Source: CAD feature listing. Evaluate the final solid. Frame: model axes, mm. Face numbers are marked on the shaded views. Round coordinates to 2 decimals unless told otherwise and drop trailing zeros. Loops run counter-clockwise (first coordinate to the right, second up) from the corner with the lowest first, then second, coordinate; pieces in that order, holes last. Notation, with made-up numbers: (-23, 86.25) -> (-13, 86.25) arc R5 ccw to (-13, 94.25) -> close; hole circle Ø11 at (47.5, 33.25). An arc over 180 degrees is marked (long way). Write item = value, one per line.
from build123d import *

# Parameters (mm, degrees)
SKETCH1_W           = 17.018
SKETCH1_H           = 7.62
BOSS_EXTRUDE1_DEPTH = 3.81
FILLET1_R           = 1.27
CUT_EXTRUDE8_REACH  = 37.332
CUT_EXTRUDE9_REACH  = 39.597
SKETCH4_R           = 1.778


with BuildPart() as part:
    # Sketch1 → Boss-Extrude1 (new body)
    with BuildSketch(Plane.XY):
        with Locations((-25.78059107, -11.13155)):
            Rectangle(SKETCH1_W, SKETCH1_H)
    extrude(amount=BOSS_EXTRUDE1_DEPTH)

    # Fillet1
    fillet1_edges = [part.edges().sort_by_distance(p)[0] for p in [
        (-17.27159107, -11.13155, 3.81),
        (-25.78059107, -14.94155, 3.81),
        (-34.28959107, -7.32155, 1.905),
        (-17.27159107, -7.32155, 1.905),
        (-17.27159107, -14.94155, 1.905),
    ]]
    fillet(fillet1_edges, radius=FILLET1_R)

    # Sketch3 → Cut-Extrude8 (cut, up to next)
    with BuildSketch(Plane.XZ.offset(14.94155), mode=Mode.PRIVATE) as cut_extrude8_sk1:
        with BuildLine():
            Line((-23.87560377, 0), (-23.87560377, 1.01854))
            ThreePointArc((-23.87560377, 1.01854), (-24.89159107, 2.0345273), (-25.90757837, 1.01854))
            Line((-25.90757837, 1.01854), (-25.90757837, 0))
            Line((-25.90757837, 0), (-23.87560377, 0))
        make_face()
    cut_extrude8_tool1 = extrude(cut_extrude8_sk1.sketch, amount=-CUT_EXTRUDE8_REACH, mode=Mode.PRIVATE) & part.part
    add(cut_extrude8_tool1.solids().sort_by_distance((-24.891591, -14.94155, 0.922401))[0], mode=Mode.SUBTRACT)

    # Sketch4 → Cut-Extrude9 (cut, up to next)
    with BuildSketch(Plane.XY.offset(3.81), mode=Mode.PRIVATE) as cut_extrude9_sk1:
        with Locations((-20.06559107, -11.13155)):
            Circle(SKETCH4_R)
    cut_extrude9_tool1 = extrude(cut_extrude9_sk1.sketch, amount=-CUT_EXTRUDE9_REACH, mode=Mode.PRIVATE) & part.part
    add(cut_extrude9_tool1.solids().sort_by_distance((-20.065591, -11.13155, 3.81))[0], mode=Mode.SUBTRACT)


solid = part.part
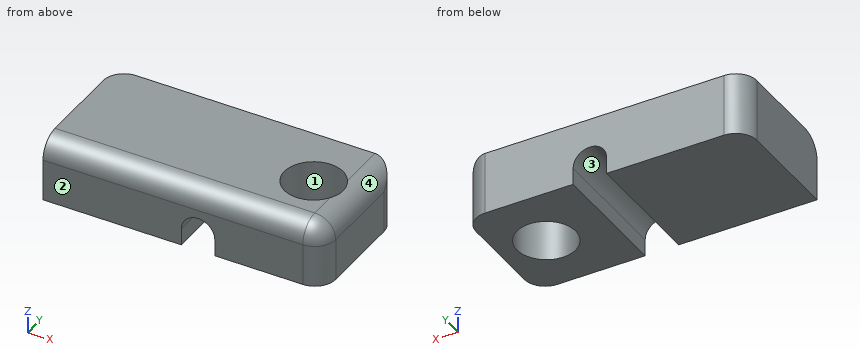
1. Mould query, pull axis X, two halves, no side actions, for the marked faces 1, 2, 3 and 4. Classes: released by +X, released by -X, zero draft, split by the parting line, or undercut.
Evaluation:
face_1 = undercut
face_2 = zero draft
face_3 = undercut
face_4 = released by +X
2. Line query: probe 1 along X at (y, z) = (-11.5, 1.25) (3 decimals); probe 2 along X at (y, z) = (-14.5, 0.4); probe 3 along X at (y, z) = (-14.5, 1.85). Output: solid intervals per line, ascending. Write a range as from..to.
Evaluation:
probe_1 = -34.29..-25.881, -23.902..-21.805, -18.326..-17.272
probe_2 = -34.29..-25.91, -23.88..-17.58
probe_3 = -34.29..-25.48, -24.31..-17.58
3. Section query B-B (y = -10.5). Return the cut outline in (x, z).
Evaluation:
outline = (-34.29, 0) -> (-25.91, 0) -> (-25.91, 1.02) arc R1.02 cw to (-23.88, 1.02) -> (-23.88, 0) -> (-21.73, 0) -> (-21.73, 3.81) -> (-34.29, 3.81) -> close; (-18.4, 0) -> (-17.27, 0) -> (-17.27, 2.54) arc R1.27 ccw to (-18.4, 3.8) -> close
4. Section query D-D (y = -13.25). Return the cut outline in (x, z), then the cut area to 3 significant figures.
Evaluation:
outline = (-34.29, 0) -> (-25.91, 0) -> (-25.91, 1.02) arc R1.02 cw to (-23.88, 1.02) -> (-23.88, 0) -> (-17.27, 0) -> (-17.27, 2.54) arc R1.27 ccw to (-18.54, 3.81) -> (-34.29, 3.81) -> close
area = 60.8 mm²
5. Section query A-A (z = 0.5). Return the cut outline in (x, y).
Evaluation:
outline = (-34.29, -14.94) -> (-25.91, -14.94) -> (-25.91, -7.32) -> (-33.02, -7.32) arc R1.27 ccw to (-34.29, -8.59) -> close; (-23.88, -14.94) -> (-18.54, -14.94) arc R1.27 ccw to (-17.27, -13.67) -> (-17.27, -8.59) arc R1.27 ccw to (-18.54, -7.32) -> (-23.88, -7.32) -> close; hole circle Ø3.56 at (-20.07, -11.13)
6. Section query C-C (x = -21.5). Return the cut outline in (y, z), then the cut area to 3 significant figures.
Evaluation:
outline = (-14.94, 0) -> (-12.18, 0) -> (-12.18, 3.81) -> (-13.67, 3.81) arc R1.27 ccw to (-14.94, 2.54) -> close; (-10.08, 0) -> (-7.32, 0) -> (-7.32, 3.81) -> (-10.08, 3.81) -> close
area = 20.7 mm²
